```python
from build123d import *

# Parameters (mm, degrees)
EXTRUDE_1_DEPTH     = 4
SKETCH_2_R          = 2.1
CUT_EXTRUDE_1_DEPTH = 4
SKETCH_3_W          = 46
SKETCH_3_H          = 2.95
EXTRUDE_2_DEPTH     = 12
FILLET_1_R          = 3
SKETCH_4_R          = 2.1
CUT_EXTRUDE_2_DEPTH = 82.469319379
CUT_EXTRUDE_3_DEPTH = 10


with BuildPart() as part:
    # 草图1 → 凸台-拉伸1 (new body)
    with BuildSketch(Plane.XY):
        with BuildLine():
            Line((-20, -45), (20, -45))
            ThreePointArc((20, -45), (22.121320344, -44.121320344), (23, -42))
            Line((23, -42), (23, 42))
            ThreePointArc((23, 42), (22.121320344, 44.121320344), (20, 45))
            Line((20, 45), (-20, 45))
            ThreePointArc((-20, 45), (-22.121320344, 44.121320344), (-23, 42))
            Line((-23, 42), (-23, -42))
            ThreePointArc((-23, -42), (-22.121320344, -44.121320344), (-20, -45))
        make_face()
    extrude(amount=EXTRUDE_1_DEPTH)

    # 草图2 → 切除-拉伸1 (cut)
    with BuildSketch(Plane.XY.offset(4)):
        with Locations((15, -37.5)):
            Circle(SKETCH_2_R)
        with Locations((-15, -37.5)):
            Circle(SKETCH_2_R)
        with Locations((-15, 37.5)):
            Circle(SKETCH_2_R)
        with Locations((15, 37.5)):
            Circle(SKETCH_2_R)
    extrude(amount=-CUT_EXTRUDE_1_DEPTH, mode=Mode.SUBTRACT)

    # 草图3 → 凸台-拉伸2 (add)
    with BuildSketch(Plane.XY.offset(4)):
        with Locations((0, 30.025)):
            Rectangle(SKETCH_3_W, SKETCH_3_H)
        with Locations((0, 21.975)):
            Rectangle(SKETCH_3_W, SKETCH_3_H)
    extrude_2 = extrude(amount=EXTRUDE_2_DEPTH)

    # 镜向1: 凸台-拉伸2 across plane
    add(extrude_2.mirror(Plane.ZX))

    # 圆角1
    fillet_1_edges = [part.edges().sort_by_distance(p)[0] for p in [
        (-23, 30.025, 16),
        (23, 30.025, 16),
        (-23, 21.975, 16),
        (23, 21.975, 16),
        (-23, -30.025, 16),
        (23, -30.025, 16),
        (23, -21.975, 16),
        (-23, -21.975, 16),
    ]]
    fillet(fillet_1_edges, radius=FILLET_1_R)

    # 草图4 → 切除-拉伸2 (cut, through all)
    with BuildSketch(Plane.XZ.offset(31.5)):
        with Locations(Location((19, 9.5, 0), (0, 0, 90))):
            Circle(SKETCH_4_R)
        with Locations(Location((-19, 9.5, 0), (0, 0, 90))):
            Circle(SKETCH_4_R)
    extrude(amount=-CUT_EXTRUDE_2_DEPTH, mode=Mode.SUBTRACT)

    # 草图5 → 切除-拉伸3 (cut)
    with BuildSketch(Plane(origin=(0, 0, 0), x_dir=(-1, 0, 0), z_dir=(0, 0, -1))):
        with BuildLine():
            Line((-5, -16), (5, -16))
            ThreePointArc((5, -16), (7.121320344, -15.121320344), (8, -13))
            Line((8, -13), (8, 13))
            ThreePointArc((8, 13), (7.121320344, 15.121320344), (5, 16))
            Line((5, 16), (-5, 16))
            ThreePointArc((-5, 16), (-7.121320344, 15.121320344), (-8, 13))
            Line((-8, 13), (-8, -13))
            ThreePointArc((-8, -13), (-7.121320344, -15.121320344), (-5, -16))
        make_face()
    extrude(amount=-CUT_EXTRUDE_3_DEPTH, mode=Mode.SUBTRACT)


solid = part.part
```
Here's how the part is built. I have some questions about the finished solid (model axes, mm). A direction names the side the tool comes from. Coordinates: 2 decimals unless noted, no trailing zeros. Order: outer loops, then holes, each group sorted by start corner. A loop starts at its lowest first (then second) coordinate and runs counter-clockwise, first axis right, second up.
1) Imagine slicing it at C-C on y = -4. List the corners of the cut face in (x, z) for me, and give its area (3 significant figures).
2) Will these pins go through, and if not, where does the flat tip stop? pin 1 (1 mm diameter, centred on x = -11.5, z = 12, fed in from +Y); pin 2 (4 mm diameter, centred on x = -19, z = 9.5, fed in from +Y) (1 decimal); pin 3 (4 mm diameter, centred on x = 10.5, y = 37, fed in from +Z); pin 4 (1 mm diameter, centred on x = -16.5, z = 5.5, fed in from -Y).
3) Which directions (+Z, -Z, +X, -X, +Y, -Y) give clear straight access to the entire face, cutting with the end or side of a thin tool? Please do faces 4 (the face through (0, 28.55, 10)), 5 (the face through (0, -38, 4)), 6 (the face through (-7.1, -15.14, 1.97)).
4) Imagine slicing it at B-B on x = 15. List the corners of the cut face in (y, z) for me.
5) Imagine slicing it at D-D on x = -6. List the corners of the cut face in (y, z) for me, and give its area (3 significant figures).
6) We'd pull the mould along X, two halves only. Please class faces 1 (the face through (-22.14, -22, 15.1)), 2 (the face through (17.581, 21.954, 7.952)), 3 (the face through (0, 26, 4)): +X half, -X half, draft (parallel to the pull), parting line (faces both ways), or undercut.
7) I need wall thicknesses on line 1 (Y direction, x = 0.5, z = 4.25); line 2 (X direction, y = 29.6, z = 9.5); line 3 (Z direction, x = 19, y = -30.45). Which ranges of each line are inside material? Lowest first, please.
8) Imagine slicing it at A-A on y = 37.5. List the corners of the cut face in (x, z) for me.
Response values:
1. outline: (-23, 0) - (-8, 0) - (-8, 4) - (-23, 4) - close; (8, 0) - (23, 0) - (23, 4) - (8, 4) - close
1. area: 120 mm2
2. pin 1: stops at y = 31.5
2. pin 2: passes through
2. pin 3: stops at z = 4
2. pin 4: stops at y = -31.5
3. face 4: +Z, +X, -X
3. face 5: +Z, +X, -X, -Y
3. face 6: +Z, -Z
4. outline: (-45, 0) - (-39.6, 0) - (-39.6, 4) - (-45, 4) - close; (-35.4, 0) - (35.4, 0) - (35.4, 4) - (31.5, 4) - (31.5, 16) - (28.55, 16) - (28.55, 4) - (23.45, 4) - (23.45, 16) - (20.5, 16) - (20.5, 4) - (-20.5, 4) - (-20.5, 16) - (-23.45, 16) - (-23.45, 4) - (-28.55, 4) - (-28.55, 16) - (-31.5, 16) - (-31.5, 4) - (-35.4, 4) - close; (39.6, 0) - (45, 0) - (45, 4) - (39.6, 4) - close
5. outline: (-45, 0) - (-15.83, 0) - (-15.83, 4) - (-20.5, 4) - (-20.5, 16) - (-23.45, 16) - (-23.45, 4) - (-28.55, 4) - (-28.55, 16) - (-31.5, 16) - (-31.5, 4) - (-45, 4) - close; (15.83, 0) - (45, 0) - (45, 4) - (31.5, 4) - (31.5, 16) - (28.55, 16) - (28.55, 4) - (23.45, 4) - (23.45, 16) - (20.5, 16) - (20.5, 4) - (15.83, 4) - close
5. area: 375 mm2
6. face 1: -X half
6. face 2: undercut
6. face 3: draft
7. line 1: y = -31.5 to -28.55, -23.45 to -20.5, 20.5 to 23.45, 28.55 to 31.5
7. line 2: x = -23 to -21.1, -16.9 to 16.9, 21.1 to 23
7. line 3: z = 0 to 7.4, 11.6 to 16
8. outline: (-23, 0) - (-17.1, 0) - (-17.1, 4) - (-23, 4) - close; (-12.9, 0) - (12.9, 0) - (12.9, 4) - (-12.9, 4) - close; (17.1, 0) - (23, 0) - (23, 4) - (17.1, 4) - close
